from build123d import *

# Parameters (mm, degrees)
SKETCH1_R           = 11.925
SKETCH1_R_2         = 9.525
BOSS_EXTRUDE1_DEPTH = 50
SKETCH2_R           = 10.85
CUT_EXTRUDE1_DEPTH  = 20
SKETCH3_R           = 10.8
CUT_EXTRUDE2_DEPTH  = 20


with BuildPart() as part:
    # Sketch1 → Boss-Extrude1 (new body)
    with BuildSketch(Plane(origin=(0, 0, 0), x_dir=(1, 0, 0), z_dir=(0, 1, 0))):
        with Locations(Location((0, 0, 0), (0, 0, 270))):
            Circle(SKETCH1_R)
        with Locations(Location((0, 0, 0), (0, 0, 270))):
            Circle(SKETCH1_R_2, mode=Mode.SUBTRACT)
    extrude(amount=BOSS_EXTRUDE1_DEPTH)

    # Sketch2 → Cut-Extrude1 (cut)
    with BuildSketch(Plane.XZ):
        with Locations(Location((0, 0, 0), (0, 0, 270))):
            Circle(SKETCH2_R)
    extrude(amount=-CUT_EXTRUDE1_DEPTH, mode=Mode.SUBTRACT)

    # Sketch3 → Cut-Extrude2 (cut)
    with BuildSketch(Plane(origin=(0, 50, 0), x_dir=(1, 0, 0), z_dir=(0, 1, 0))):
        with Locations(Location((0, 0, 0), (0, 0, 270))):
            Circle(SKETCH3_R)
    extrude(amount=-CUT_EXTRUDE2_DEPTH, mode=Mode.SUBTRACT)


solid = part.part
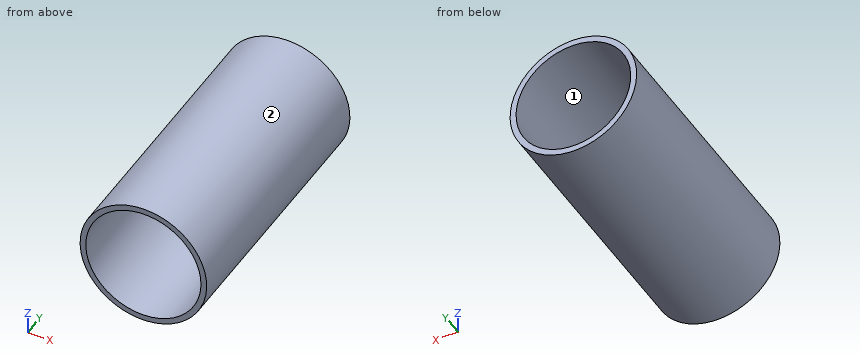
Could you check a few things on this model? Use its own coordinates, in mm. Face numbers are marked on the shaded views. Give positions to 0.01 mm unless a question says otherwise; leave off trailing zeros. Order: outer loops, then holes, each group sorted by start corner. A loop starts at its lowest first (then second) coordinate and runs counter-clockwise, first axis right, second up. Notation, with made-up numbers: M 66,29.5 L 113,29.5 A13 ccw 113,36.5 Z; hole C 5,33 d2. An arc over 180 degrees is marked long. One line per question, with ' | ' between items.
1. If I drill on line 1 (X direction, y = 44.25, z = 0) (3 decimals); line 2 (Z direction, x = -3.5, y = 40.5); line 3 (X direction, y = 17.5, z = 9.25), over which ranges is the centre line in solid material (lowest first)?
Results:
line 1: -11.925 to -10.8, 10.8 to 11.925 | line 2: -11.4 to -10.22, 10.22 to 11.4 | line 3: -7.53 to -5.67, 5.67 to 7.53
2. I want a section at D-D (y = 44.5). List the corners of the cut face in (x, z) for me (3 decimals).
Results:
outline: C 0,0 d23.85; hole C 0,0 d21.6
3. I want a section at A-A (x = 0). List the corners of the cut face in (y, z) for me (3 decimals), and give its area (3 significant figures).
Results:
outline: M 0,-11.925 L 50,-11.925 L 50,-10.8 L 30,-10.8 L 30,-9.525 L 20,-9.525 L 20,-10.85 L 0,-10.85 Z; M 0,10.85 L 20,10.85 L 20,9.525 L 30,9.525 L 30,10.8 L 50,10.8 L 50,11.925 L 0,11.925 Z | area: 136 mm²
4. I want a section at C-C (y = 13.5). List the corners of the cut face in (x, z) for me (3 decimals), and give its area (3 significant figures).
Results:
outline: C 0,0 d23.85; hole C 0,0 d21.7 | area: 76.9 mm²
5. We'd pull the mould along X, two halves only. Please class the marked faces 1 and 2: +X half, -X half, draft (parallel to the pull), parting line (faces both ways), or undercut.
Results:
face 1: undercut | face 2: parting line
6. I want a section at B-B (z = 9). List the corners of the cut face in (x, y) for me.
Results:
outline: M -7.82,0 L -6.06,0 L -6.06,20 L -3.12,20 L -3.12,30 L -5.97,30 L -5.97,50 L -7.82,50 Z; M 3.12,20 L 6.06,20 L 6.06,0 L 7.82,0 L 7.82,50 L 5.97,50 L 5.97,30 L 3.12,30 Z
7. I'm going to push flat-ended pins straight in: pin 1 (1.5 mm diameter, centred on x = -6, z = -7.5, fed in from -Y); pin 2 (1.5 mm diameter, centred on y = 15.5, z = -5.5, fed in from -X); pin 3 (12 mm diameter, centred on x = 7.5, y = 25, fed in from -Z); pin 4 (11.5 mm diameter, centred on x = 0, z = 0, fed in from -Y). Where does each tip first touch, or does it pass through?
Results:
pin 1: y = 20 | pin 2: x = -10.94 | pin 3: z = -11.83 | pin 4: through
